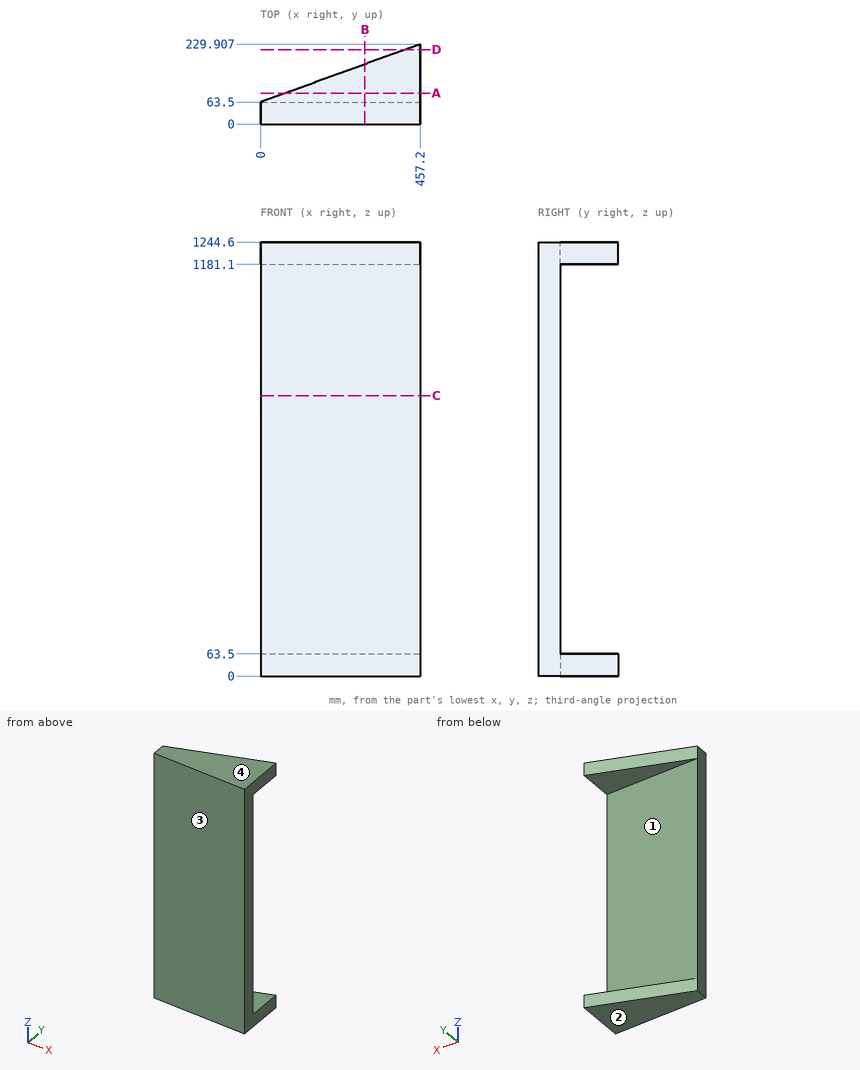
Input: dimensioned drawing with shaded views. Units: mm. Origin: part minimum x, y, z. Coordinates: 2 decimals unless noted, no trailing zeros. Write each loop counter-clockwise with the first axis right and the second up, starting at its lowest first coordinate (ties: lowest second). Pieces come first, ordered by that corner, then holes. Notation, with made-up numbers: M 27,60.5 L 79,60.5 A34 cw 79,90.5 Z; hole C 88.5,21.25 d11. An arc over 180 degrees is marked long. Use one line per item in the form item = value.
Q1. Section B-B (x = 298.5). Return loops of the section in (y, z) (1 decimal).
Answer below:
outline = M 0,0 L 172.1,0 L 172.1,63.5 L 63.5,63.5 L 63.5,1181.1 L 172.1,1181.1 L 172.1,1244.6 L 0,1244.6 Z
Q2. First-contact query: pin 1 (12 mm diameter, centred on x = 171, z = 888, fed in from +Y). Flat tip, straight axial feed; report the tip coordinate or a pass-through.
Answer below:
pin_1 = 63.5
Q3. Section D-D (y = 213.5). Return loops of the section in (x, z), plus the area to 4 significant figures.
Answer below:
outline = M 412.12,0 L 457.2,0 L 457.2,63.5 L 412.12,63.5 Z; M 412.12,1181.1 L 457.2,1181.1 L 457.2,1244.6 L 412.12,1244.6 Z
area = 5,725 mm²
Q4. Section C-C (z = 804.5). Return loops of the section in (x, y).
Answer below:
outline = M 0,0 L 457.2,0 L 457.2,63.5 L 0,63.5 Z
Q5. Section A-A (y = 89). Return loops of the section in (x, z).
Answer below:
outline = M 70.06,0 L 457.2,0 L 457.2,63.5 L 70.06,63.5 Z; M 70.06,1181.1 L 457.2,1181.1 L 457.2,1244.6 L 70.06,1244.6 Z
Q6. Draft query along Z for the marked faces 1, 2, 3 and 4. Return one class per face: released by +Z, released by -Z, zero draft, split by the parting line, or undercut.
Answer below:
face_1 = undercut
face_2 = released by -Z
face_3 = zero draft
face_4 = released by +Z
Q7. Material intervals for probe 1 along Z at (x, y) = (428, 163); probe 2 along Y at (x, z) = (167.5, 709), sorted ascending. Write a range as from..to.
Answer below:
probe_1 = 0..63.5, 1181.1..1244.6
probe_2 = 0..63.5
